```python
from build123d import *

# Parameters (mm, degrees)
BOSS_EXTRUDE2_DEPTH      = 12
BOSS_EXTRUDE2_DEPTH_BACK = 12
SKETCH1_R                = 7.625
SKETCH1_R_2              = 5
FILLET1_R                = 10
CUT_EXTRUDE1_START       = -7
SKETCH2_R                = 5
CUT_EXTRUDE1_DEPTH       = 7
SKETCH3_R                = 5
CUT_EXTRUDE2_DEPTH       = 7


with BuildPart() as part:
    # Sketch1 → Boss-Extrude2 (new, two sides: drawn at the far end of the back side and taken through both)
    with BuildSketch(Plane(origin=(0, 0, 0), x_dir=(0, 0, -1), z_dir=(1, 0, 0)).offset(-BOSS_EXTRUDE2_DEPTH_BACK)):
        with BuildLine():
            ThreePointArc((-10.249331942, 5.817161927), (0, -11.785082866), (10.249331942, 5.817161927))
            ThreePointArc((10.249331942, 5.817161927), (4.569540082, 31.759611334), (7.275406493, 58.178335825))
            ThreePointArc((7.275406493, 58.178335825), (0, 67.5), (-7.275406493, 58.178335825))
            ThreePointArc((-7.275406493, 58.178335825), (-4.569540082, 31.759611334), (-10.249331942, 5.817161927))
        make_face()
        Circle(SKETCH1_R, mode=Mode.SUBTRACT)
        with Locations((0, 60)):
            Circle(SKETCH1_R_2, mode=Mode.SUBTRACT)
    extrude(amount=BOSS_EXTRUDE2_DEPTH + BOSS_EXTRUDE2_DEPTH_BACK)

    # Fillet1
    fillet1_edges = [part.edges().sort_by_distance(p)[0] for p in [
        (0, 5.817161927, -10.249331942),
        (0, 5.817161927, 10.249331942),
    ]]
    fillet(fillet1_edges, radius=FILLET1_R)

    # Sketch2 → Cut-Extrude1 (cut)
    # profile 1 of 2: a face of its own
    with BuildSketch(Plane(origin=(12, 0, 0), x_dir=(0, 0, -1), z_dir=(1, 0, 0)).offset(CUT_EXTRUDE1_START)):
        with BuildLine():
            ThreePointArc((7.220530461, 57.971715045), (0, 52.5), (-7.220530461, 57.971715045))
            ThreePointArc((-7.220530461, 57.971715045), (-4.557224249, 31.98164601), (-10.010939305, 6.431031917))
            ThreePointArc((-10.010939305, 6.431031917), (-10.224413054, 5.917964178), (-10.466057682, 5.417546931))
            ThreePointArc((-10.466057682, 5.417546931), (0, 11.785082866), (10.466057682, 5.417546931))
            ThreePointArc((10.466057682, 5.417546931), (10.224413054, 5.917964178), (10.010939305, 6.431031917))
            ThreePointArc((10.010939305, 6.431031917), (4.557224249, 31.98164601), (7.220530461, 57.971715045))
        make_face()
    # profile 2 of 2: a face of its own
    with BuildSketch(Plane(origin=(12, 0, 0), x_dir=(0, 0, -1), z_dir=(1, 0, 0)).offset(CUT_EXTRUDE1_START)):
        with BuildLine():
            ThreePointArc((7.275406493, 58.178335825), (7.443639859, 59.082271471), (7.5, 60))
            ThreePointArc((7.5, 60), (-0.917728529, 67.443639859), (-7.275406493, 58.178335825))
            ThreePointArc((-7.275406493, 58.178335825), (-7.24790272, 58.075042899), (-7.220530461, 57.971715045))
            ThreePointArc((-7.220530461, 57.971715045), (0, 52.5), (7.220530461, 57.971715045))
            ThreePointArc((7.220530461, 57.971715045), (7.24790272, 58.075042899), (7.275406493, 58.178335825))
        make_face()
        with Locations((0, 60)):
            Circle(SKETCH2_R, mode=Mode.SUBTRACT)
    extrude(amount=CUT_EXTRUDE1_DEPTH, mode=Mode.SUBTRACT)

    # Sketch3 → Cut-Extrude2 (cut)
    # profile 1 of 2: a face of its own
    with BuildSketch(Plane.ZY.offset(12)):
        with BuildLine():
            ThreePointArc((7.220530461, 57.971715045), (0, 52.5), (-7.220530461, 57.971715045))
            ThreePointArc((-7.220530461, 57.971715045), (-4.557224249, 31.98164601), (-10.010939305, 6.431031917))
            ThreePointArc((-10.010939305, 6.431031917), (-10.224413054, 5.917964178), (-10.466057682, 5.417546931))
            ThreePointArc((-10.466057682, 5.417546931), (0, 11.785082866), (10.466057682, 5.417546931))
            ThreePointArc((10.466057682, 5.417546931), (10.224413054, 5.917964178), (10.010939305, 6.431031917))
            ThreePointArc((10.010939305, 6.431031917), (4.557224249, 31.98164601), (7.220530461, 57.971715045))
        make_face()
    # profile 2 of 2: a face of its own
    with BuildSketch(Plane.ZY.offset(12)):
        with BuildLine():
            ThreePointArc((7.275406493, 58.178335825), (7.443639859, 59.082271471), (7.5, 60))
            ThreePointArc((7.5, 60), (-0.917728529, 67.443639859), (-7.275406493, 58.178335825))
            ThreePointArc((-7.275406493, 58.178335825), (-7.24790272, 58.075042899), (-7.220530461, 57.971715045))
            ThreePointArc((-7.220530461, 57.971715045), (0, 52.5), (7.220530461, 57.971715045))
            ThreePointArc((7.220530461, 57.971715045), (7.24790272, 58.075042899), (7.275406493, 58.178335825))
        make_face()
        with Locations((0, 60)):
            Circle(SKETCH3_R, mode=Mode.SUBTRACT)
    extrude(amount=-CUT_EXTRUDE2_DEPTH, mode=Mode.SUBTRACT)


solid = part.part
```
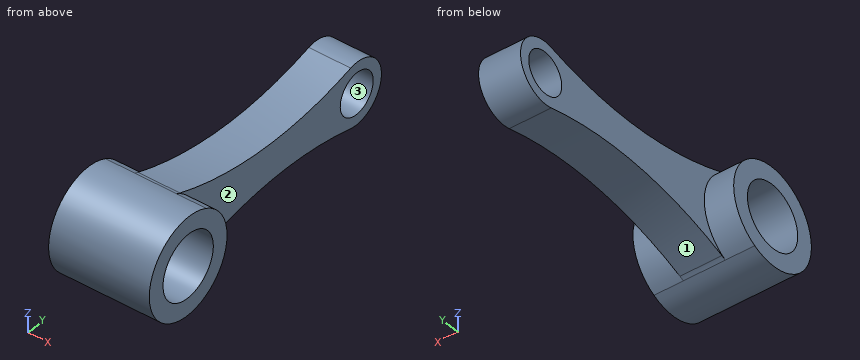
Could you check a few things on this model? Use its own coordinates, in mm. Face numbers are marked on the shaded views. Round coordinates to 2 decimals unless told otherwise and drop trailing zeros. Loops run counter-clockwise (first coordinate to the right, second up) from the corner with the lowest first, then second, coordinate; pieces in that order, holes last. Notation, with made-up numbers: M 2.5,27 L 27.5,27 A38 ccw 27.5,65 Z; hole C 3.5,-14.75 d11. An arc over 180 degrees is marked long. Answer as CSV lines item,"result".
1) Imagine slicing it at C-C on y = 60. List the corners of the cut face in (x, z) for me, and give its area (3 significant figures).
From the geometry:
outline,"M -5,-7.5 L 5,-7.5 L 5,-5 L -5,-5 Z; M -5,5 L 5,5 L 5,7.5 L -5,7.5 Z"
area,"50.0 mm^2"
2) We'd pull the mould along Z, two halves only. Please class the marked faces 1, 2 and 3: released by +Z, released by -Z, zero draft, split by the parting line, or undercut.
From the geometry:
face 1,"released by -Z"
face 2,"zero draft"
face 3,"undercut"
3) Imagine slicing it at B-B on z = 0. List the corners of the cut face in (x, y) for me (3 decimals).
From the geometry:
outline,"M -12,-11.785 L 12,-11.785 L 12,-7.625 L -12,-7.625 Z; M -12,7.625 L 12,7.625 L 12,11.785 L 5,11.785 L 5,55 L -5,55 L -5,11.785 L -12,11.785 Z; M -5,65 L 5,65 L 5,67.5 L -5,67.5 Z"
4) If I drill on probe 1 along Y at (x, z) = (-2.5, 0) (3 decimals); probe 2 along Y at (x, z) = (0, -0.75); probe 3 along Z at (x, y) = (9, -2.5), over which ranges is the centre line in solid material (lowest first)?
From the geometry:
probe 1,"-11.785 to -7.625, 7.625 to 55, 65 to 67.5"
probe 2,"-11.76 to -7.59, 7.59 to 55.06, 64.94 to 67.46"
probe 3,"-11.52 to -7.2, 7.2 to 11.52"
5) Imagine slicing it at D-D on z = -8.5. List the corners of the cut face in (x, y) for me, and give its area (3 significant figures).
From the geometry:
outline,"M -12,-8.16 L 12,-8.16 L 12,8.16 L 5,8.16 L 5,10.71 L -5,10.71 L -5,8.16 L -12,8.16 Z"
area,"417 mm^2"
6) Imagine slicing it at A-A on y = 0. List the corners of the cut face in (x, z) for me (3 decimals).
From the geometry:
outline,"M -12,-11.785 L 12,-11.785 L 12,-7.625 L -12,-7.625 Z; M -12,7.625 L 12,7.625 L 12,11.785 L -12,11.785 Z"
7) For pin 1 Ø8 at (x, z) = (2.5, 9.5) entering from +Y; pin 2 Ø2 at (y, z) = (22.5, -6.5) entering from +X; pin 3 Ø4 at (x, z) = (1.5, 3) entering from -Y; pin 4 Ø12 at (y, z) = (0, 0) entering from +X, each with a flat end and sliding along its axis, tell me the tip position at first contact or that it passes through.
From the geometry:
pin 1,"y = 65.1"
pin 2,"x = 5"
pin 3,"y = -11.74"
pin 4,"through"
